Design review of the part built by this model. Coordinates are the model's own, in mm. Face numbers are marked on the shaded views. A direction names the side the tool comes from. Coordinates: 2 decimals unless noted, no trailing zeros. Write each loop counter-clockwise with the first axis right and the second up, starting at its lowest first coordinate (ties: lowest second). Pieces come first, ordered by that corner, then holes. Notation, with made-up numbers: (64.5, 20) - (99.5, 20) arc R20 cw to (99.5, 43) - close; hole circle Ø4 at (63.5, -3.5). An arc over 180 degrees is marked (long way). Use a Markdown table: item, result.
Autodesk Inventor part; units mm, degrees
ref_plane "YZ Plane" through (0, 0, 0) normal (1, 0, 0) x (0, 1, 0)
ref_plane "XZ Plane" through (0, 0, 0) normal (0, 1, 0) x (-1, 0, 0)
ref_plane "XY Plane" through (0, 0, 0) normal (0, 0, 1) x (1, 0, 0)
sketch "Sketch1" plane through (0, 0, 0) normal (0, 1, 0) x (-1, 0, 0)
  line L0 (0, 0) -> (5, 0)
  line L1 (5, 0) -> (5, -15)
  line L2 (5, -15) -> (0, -15)
  line L3 (0, -15) -> (0, 0)
  line L4 (0, 0) -> (-10, 0)
  line L5 (-10, 0) -> (-10, -5)
  line L6 (-10, -5) -> (0, -5)
  line L7 (0, -5) -> (0, 0)
  dimension "d0" = 5
  dimension "d1" = 5
  dimension "d2" = 15
  dimension "d3" = 10
extrude "Extrusion1" add sketch "Sketch1" along normal blind 15
sketch "Sketch2" plane through (0, 15, 0) normal (0, 1, 0) x (1, 0, 0)
  circle A0 centre (-2, 3) radius 1.5
  line L0 (-5, 15) -> (-5, 0)
  line L1 (-5, 0) -> (10, 0)
  point P0 (0, 0)
  dimension "d6" = 3
  dimension "d7" = 3
  dimension "d8" = 3
fillet "Fillet1" radius 4 1 edges at (-5, 7.5, 0)
extrude "Extrusion2" cut sketch "Sketch2" against normal blind 10
properties part number "CornerTest01"
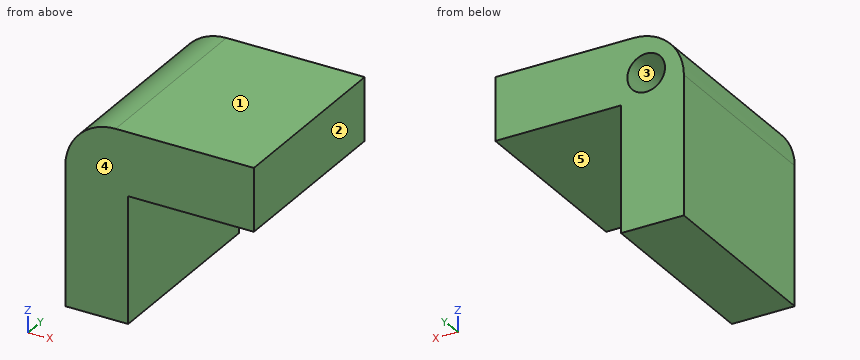
(1) For L1, parallel to X at y = 4, z = -11.5; L2, parallel to Z at x = -2, y = 8.25, list the stretches that pass through material, from the lowest coordinate up. Write a range as from..to.
Determined:
| item | result |
|---|---|
| L1 | -5..0 |
| L2 | -15..-4.5, -1.5..-0.13 |
(2) Take a section at D-D on z = -11.5. Write out the cut boundary in (x, y), and give its area (3 significant figures).
Determined:
| item | result |
|---|---|
| outline | (-5, 0) - (0, 0) - (0, 15) - (-5, 15) - close |
| area | 75.0 mm2 |
(3) Take a section at C-C on x = 5.75. Write out the cut boundary in (y, z).
Determined:
| item | result |
|---|---|
| outline | (0, -5) - (15, -5) - (15, 0) - (0, 0) - close |
(4) Take a section at A-A on y = 12.5. Write out the cut boundary in (x, z).
Determined:
| item | result |
|---|---|
| outline | (-5, -15) - (0, -15) - (0, -5) - (10, -5) - (10, 0) - (-1, 0) arc R4 ccw to (-5, -4) - close; hole circle Ø3 at (-2, -3) |
(5) Draft analysis for pull direction Z (two halves, no side actions). For the marked faces 1, 2 and 3, state which applies: +Z half, -Z half, draft (parallel to the pull), parting line (faces both ways), or undercut.
Determined:
| item | result |
|---|---|
| face 1 | +Z half |
| face 2 | draft |
| face 3 | undercut |
(6) Machinability: for the marked faces 4 and 5, which of the approach directions +Z, -Z, +X, -X, +Y, -Y give a long, thin tool a straight path to every point of the face, cutting with its end or side? Answer none if there is none.
Determined:
| item | result |
|---|---|
| face 4 | +Z, -Z, +X, -X, -Y |
| face 5 | -Z, +X, +Y, -Y |
(7) For pin 1 (8 mm diameter, centred on x = 1.5, y = 5.5, fed in from +Z); pin 2 (2 mm diameter, centred on x = 6, y = 2.5, fed in from -Z); pin 3 (8 mm diameter, centred on y = 11, z = -10.5, fed in from +X); pin 4 (1.5 mm diameter, centred on x = -2.5, z = -3, fed in from +Y), all flat-tipped, find the tip position at first contact; note any pin that passes through.
Determined:
| item | result |
|---|---|
| pin 1 | z = 0 |
| pin 2 | z = -5 |
| pin 3 | x = 0 |
| pin 4 | y = 5 |
(8) Take a section at B-B on y = 3. Write out the cut boundary in (x, z).
Determined:
| item | result |
|---|---|
| outline | (-5, -15) - (0, -15) - (0, -5) - (10, -5) - (10, 0) - (-1, 0) arc R4 ccw to (-5, -4) - close |
